Could you check a few things on this model? Use its own coordinates, in mm. A direction names the side the tool comes from. Round coordinates to 2 decimals unless told otherwise and drop trailing zeros. Write each loop counter-clockwise with the first axis right and the second up, starting at its lowest first coordinate (ties: lowest second). Pieces come first, ordered by that corner, then holes. Notation, with made-up numbers: (88.25, 55) - (127.25, 55) arc R9 cw to (127.25, 71) - close; hole circle Ø8 at (23.5, 36). An arc over 180 degrees is marked (long way). Put each result on its own line as item: value.
from build123d import *

# Parameters (mm, degrees)
SKETCH_1_R      = 7.5
EXTRUDE_1_DEPTH = 170


with BuildPart() as part:
    # 草图1 → 凸台-拉伸1 (new body)
    with BuildSketch(Plane.XY):
        with BuildLine():
            Line((0, -10), (-110, -10))
            Line((-110, -10), (-220.810216861, 91.099435405))
            Line((-220.810216861, 91.099435405), (-177.785501138, 141.099435405))
            Line((-177.785501138, 141.099435405), (-155.045503197, 121.531796466))
            Line((-155.045503197, 121.531796466), (-174.921114521, 98.433896817))
            Line((-174.921114521, 98.433896817), (-77.942720008, 9.954140983))
            Line((-77.942720008, 9.954140983), (-0.956596724, 9.954140983))
            ThreePointArc((-0.956596724, 9.954140983), (9.988528666, 0.478847664), (0, -10))
        make_face()
        Circle(SKETCH_1_R, mode=Mode.SUBTRACT)
    extrude(amount=EXTRUDE_1_DEPTH)


solid = part.part
(1) Imagine slicing it at C-C, the plane x = -36.5. List the corners of the cut face in (y, z) for me, then the cut area to 3 significant figures.
Values found:
outline: (-10, 0) - (9.95, 0) - (9.95, 170) - (-10, 170) - close
area: 3,390 mm^2
(2) Please list where these lines run through material, in increasing order: probe 1 along Y at (x, z) = (-62, 126.5); probe 2 along X at (y, z) = (-1, 152.5); probe 3 along Y at (x, z) = (-111, 81.5). Write a range as from..to.
Values found:
probe 1: y = -10..9.95
probe 2: x = -119.86..-7.43, 7.43..9.95
probe 3: y = -9.09..40.11
(3) For faces 4 (the face through (-164.63, 39.84, 83.81)), 5 (the face through (-164.844, 110.145, 83.81)), which set-ups out of +Z, -Z, +X, -X, +Y, -Y let a thin tool reach every point of the face, with its end or its side?
Values found:
face 4: +Z, -Z, -X, -Y
face 5: +Z, -Z, +X
(4) Imagine slicing it at A-A, the plane z = 130.5. List the corners of the cut face in (x, y) for me, then the cut area to 3 significant figures.
Values found:
outline: (-220.81, 91.1) - (-110, -10) - (0, -10) arc R10 ccw (long way) to (-0.96, 9.95) - (-77.94, 9.95) - (-174.92, 98.43) - (-155.05, 121.53) - (-177.79, 141.1) - close; hole circle Ø15 at (0, 0)
area: 8,410 mm^2
(5) I'm going to push flat-ended pins straight in: pin 1 (23 mm diameter, centred on x = -21.5, z = 62.5, fed in from +Y); pin 2 (6 mm diameter, centred on y = 18.5, z = 149.5, fed in from +X); pin 3 (8 mm diameter, centred on y = 86.5, z = 40, fed in from +X). Where does each tip first touch, or does it pass through?
Values found:
pin 1: stops at y = 9.95
pin 2: stops at x = -84.02
pin 3: stops at x = -157.46
(6) Imagine slicing it at B-B, the plane y = 0. List the corners of the cut face in (x, z) for me.
Values found:
outline: (-120.96, 0) - (-7.5, 0) - (-7.5, 170) - (-120.96, 170) - close; (7.5, 0) - (10, 0) - (10, 170) - (7.5, 170) - close
(7) Imagine slicing it at D-D, the plane y = 102. List the corners of the cut face in (x, z) for me, then the cut area to 3 significant figures.
Values found:
outline: (-211.43, 0) - (-171.85, 0) - (-171.85, 170) - (-211.43, 170) - close
area: 6,730 mm^2
(8) If we mould it in two halves opening along Y, with no side actions, what happens to faces 1 (the face through (-127.11, 54.81, 83.81)), 2 (the face through (-131, 44, 170)), 3 (the face through (-166.57, 131.45, 83.81))? For each: pulls with the +Y half, pulls with the -Y half, needs draft (parallel to the pull), parting line crosses it, or undercut.
Values found:
face 1: undercut
face 2: needs draft
face 3: pulls with the +Y half
